Read the model definition and answer for the solid it produces. Units are mm, in the model's axes. A direction names the side the tool comes from. Coordinates: 2 decimals unless noted, no trailing zeros. Loops run counter-clockwise (first coordinate to the right, second up) from the corner with the lowest first, then second, coordinate; pieces in that order, holes last. Notation, with made-up numbers: (73.25, 8) -> (105.25, 8) arc R19 ccw to (105.25, 40) -> close; hole circle Ø10 at (36.25, 22). An arc over 180 degrees is marked (long way). Answer as a JSON object with one key per item and string values. Group by question number.
1) Flat-ended cylindrical pins translate along their axes: P1, Ø8, axis at x = 35, z = -6, coming from the +Y side; P2, Ø6.5, axis at x = 29.5, y = 8.5, coming from the +Z side; P3, Ø3.5, axis at y = 7, z = -9.5, coming from the -X side; P4, Ø5, axis at x = 8, y = 10, coming from the -Z side. Find the tip coordinate at first contact, or state that the pin passes through.
2) Section D-D, the plane x = 7 is taken. Give the vertices of the cut face in (y, z).
3) Determine the mould class of faces 4 (the face through (30, 6, -13)), 5 (the face through (32, 6, -17.5)), 6 (the face through (32, 4, -2.5)) for opening direction Z: released by +Z, released by -Z, zero draft, split by the parting line, or undercut.
4) Consider probe 1 along X at (y, z) = (0.4, -18.5); probe 2 along X at (y, z) = (5.5, -12); probe 3 along X at (y, z) = (0.4, -2.5). Determine where each line is inside the solid, lowest interval first. Write a range as [from, to].
5) Section B-B, the plane z = -18.5 is taken. Give the vertices of the cut face in (x, y).
6) Section C-C, the plane x = 40.5 is taken. Give the vertices of the cut face in (y, z).
7) Which of the six approach directions +Z, -Z, +X, -X, +Y, -Y give full straight-line access (tool end or side, diameter ignored) to faces 1 (the face through (21, 5, -16.5)), 2 (the face through (36.5, 6, -16)), 3 (the face through (29, 4, -11))?
8) Section A-A, the plane y = 5 is taken. Give the vertices of the cut face in (x, z).
from build123d import *

# Parameters (mm, degrees)
SKETCH1_W               = 43
SKETCH1_H               = 21
PCB_DEPTH               = 1.6
MOUNT_HOLE_1_DEPTH      = 48.880685041
MOUNT_HOLE_1_DEPTH_BACK = 48.880685041
SKETCH2_R               = 1.5
MOUNT_HOLE_2_DEPTH      = 48.880685041
MOUNT_HOLE_2_DEPTH_BACK = 48.880685041
SKETCH3_R               = 1.5
INDUCTOR_START          = 1.6
SKETCH4_W               = 12
SKETCH4_H               = 12
INDUCTOR_DEPTH          = 7
CAP_IN_START            = 1.6
SKETCH5_R               = 4
CAP_IN_DEPTH            = 12
CAP_OUT_START           = 1.6
SKETCH6_R               = 4
CAP_OUT_DEPTH           = 12
TRIM_POT_START          = 1.6
SKETCH7_W               = 9.5
SKETCH7_H               = 4.5
TRIM_POT_DEPTH          = 9.5
LM2596S_START           = 1.6
SKETCH8_W               = 10
SKETCH8_H               = 8.5
LM2596S_DEPTH           = 4.5


with BuildPart() as part:
    # Sketch1 → PCB (new body)
    with BuildSketch(Plane(origin=(0, 0, 0), x_dir=(1, 0, 0), z_dir=(0, 1, 0))):
        with Locations((21.5, 10.5)):
            Rectangle(SKETCH1_W, SKETCH1_H)
    extrude(amount=PCB_DEPTH)

    # Sketch2 → Mount_hole_1 (cut, two sides: drawn at the far end of the back side and taken through both)
    with BuildSketch(Plane(origin=(0, 0, 0), x_dir=(1, 0, 0), z_dir=(0, 1, 0)).offset(-MOUNT_HOLE_1_DEPTH_BACK)):
        with Locations(Location((2.5, 2.5, 0), (0, 0, 270))):
            Circle(SKETCH2_R)
    extrude(amount=MOUNT_HOLE_1_DEPTH + MOUNT_HOLE_1_DEPTH_BACK, mode=Mode.SUBTRACT)

    # Sketch3 → Mount_hole_2 (cut, two sides: drawn at the far end of the back side and taken through both)
    with BuildSketch(Plane(origin=(0, 0, 0), x_dir=(1, 0, 0), z_dir=(0, 1, 0)).offset(-MOUNT_HOLE_2_DEPTH_BACK)):
        with Locations(Location((40.5, 18.5, 0), (0, 0, 270))):
            Circle(SKETCH3_R)
    extrude(amount=MOUNT_HOLE_2_DEPTH + MOUNT_HOLE_2_DEPTH_BACK, mode=Mode.SUBTRACT)

    # Sketch4 → Inductor (add)
    with BuildSketch(Plane(origin=(0, 0, 0), x_dir=(1, 0, 0), z_dir=(0, 1, 0)).offset(INDUCTOR_START)):
        with Locations((21, 10.5)):
            Rectangle(SKETCH4_W, SKETCH4_H)
    extrude(amount=INDUCTOR_DEPTH)

    # Sketch5 → Cap_in (add)
    with BuildSketch(Plane(origin=(0, 0, 0), x_dir=(1, 0, 0), z_dir=(0, 1, 0)).offset(CAP_IN_START)):
        with Locations(Location((7, 10.5, 0), (0, 0, 90))):
            Circle(SKETCH5_R)
    extrude(amount=CAP_IN_DEPTH)

    # Sketch6 → Cap_out (add)
    with BuildSketch(Plane(origin=(0, 0, 0), x_dir=(1, 0, 0), z_dir=(0, 1, 0)).offset(CAP_OUT_START)):
        with Locations(Location((36, 10.5, 0), (0, 0, 90))):
            Circle(SKETCH6_R)
    extrude(amount=CAP_OUT_DEPTH)

    # Sketch7 → Trim_pot (add)
    with BuildSketch(Plane(origin=(0, 0, 0), x_dir=(1, 0, 0), z_dir=(0, 1, 0)).offset(TRIM_POT_START)):
        with Locations((31.75, 15.25)):
            Rectangle(SKETCH7_W, SKETCH7_H)
    extrude(amount=TRIM_POT_DEPTH)

    # Sketch8 → LM2596S (add)
    with BuildSketch(Plane(origin=(0, 0, 0), x_dir=(1, 0, 0), z_dir=(0, 1, 0)).offset(LM2596S_START)):
        with Locations((32, 6.75)):
            Rectangle(SKETCH8_W, SKETCH8_H)
    extrude(amount=LM2596S_DEPTH)


solid = part.part
Determined:
{
 "1": {"P1": "y = 13.6", "P2": "z = -2.5", "P3": "x = 3", "P4": "z = -14.5"},
 "2": {"outline": "(0, -21) -> (1.6, -21) -> (1.6, -14.5) -> (13.6, -14.5) -> (13.6, -6.5) -> (1.6, -6.5) -> (1.6, 0) -> (0, 0) -> close"},
 "3": {"face 4": "undercut", "face 5": "released by -Z", "face 6": "released by +Z"},
 "4": {"probe 1": "[0, 39], [42, 43]", "probe 2": "[3.29, 10.71], [15, 27], [32.29, 39.71]", "probe 3": "[0, 1], [4, 43]"},
 "5": {"outline": "(0, 0) -> (39, 0) -> (39, 1.6) -> (0, 1.6) -> close; (42, 0) -> (43, 0) -> (43, 1.6) -> (42, 1.6) -> close"},
 "6": {"outline": "(0, -21) -> (1.6, -21) -> (1.6, -20) -> (0, -20) -> close; (0, -17) -> (1.6, -17) -> (1.6, 0) -> (0, 0) -> close"},
 "7": {"face 1": "-Z, -X, +Y", "face 2": "-Z, +X, +Y", "face 3": "+Y"},
 "8": {"outline": "circle Ø8 at (7, -10.5); (15, -16.5) -> (27, -16.5) -> (27, -17.5) -> (36.5, -17.5) -> (36.5, -14.47) arc R4 ccw to (37, -6.63) -> (37, -2.5) -> (27, -2.5) -> (27, -4.5) -> (15, -4.5) -> close; hole (27, -13) -> (32.88, -13) arc R4 cw to (32.03, -11) -> (27, -11) -> close"}
}
